```python
from build123d import *

# Parameters (mm, degrees)
BOSS_EXTRUDE1_DEPTH = 200.8
CUT_EXTRUDE3_DEPTH  = 36.191113799
SKETCH5_W           = 20
SKETCH5_H           = 5
SKETCH5_W_2         = 3
SKETCH5_H_2         = 20
SKETCH5_H_3         = 3
BOSS_EXTRUDE2_DEPTH = 5


with BuildPart() as part:
    # Sketch2 → Boss-Extrude1 (new body)
    with BuildSketch(Plane.XY.offset(2)):
        Polygon((22.534227339, 12.285835046), (24.243029584, 7.58689954), (-64.096957923, -24.53858267), (-65.805760168, -19.839647165), align=None)
    extrude(amount=BOSS_EXTRUDE1_DEPTH)

    # Sketch4 → Cut-Extrude3 (cut, through all)
    with BuildSketch(Plane(origin=(0.394814778, -1.085678102, 0), x_dir=(-0.939787101, -0.341760449, 0), z_dir=(0.341760449, -0.939787101, 0))):
        Polygon((19.52381131, -2), (23.72381131, -2), (23.72381131, -6), (25.42381131, -6), (25.42381131, -8.8), (23.72381131, -8.8), (23.72381131, -18.8), (19.52381131, -18.8), (19.52381131, -8.8), (17.82381131, -8.8), (17.82381131, -6), (19.52381131, -6), align=None)
        Polygon((-25.37618869, -54.3), (-25.37618869, -50.1), (-21.37618869, -50.1), (-21.37618869, -48.4), (-18.57618869, -48.4), (-18.57618869, -50.1), (-8.57618869, -50.1), (-8.57618869, -54.3), (-18.57618869, -54.3), (-18.57618869, -56), (-21.37618869, -56), (-21.37618869, -54.3), align=None)
        Polygon((23.72381131, -202.8), (19.52381131, -202.8), (19.52381131, -198.8), (17.82381131, -198.8), (17.82381131, -196), (19.52381131, -196), (19.52381131, -186), (23.72381131, -186), (23.72381131, -196), (25.42381131, -196), (25.42381131, -198.8), (23.72381131, -198.8), align=None)
        Polygon((-21.37618869, -154.7), (-21.37618869, -156.4), (-18.57618869, -156.4), (-18.57618869, -154.7), (-8.57618869, -154.7), (-8.57618869, -150.5), (-18.57618869, -150.5), (-18.57618869, -148.8), (-21.37618869, -148.8), (-21.37618869, -150.5), (-25.37618869, -150.5), (-25.37618869, -154.7), align=None)
        Polygon((68.62381131, -150.5), (68.62381131, -154.7), (64.62381131, -154.7), (64.62381131, -156.4), (61.82381131, -156.4), (61.82381131, -154.7), (51.82381131, -154.7), (51.82381131, -150.5), (61.82381131, -150.5), (61.82381131, -148.8), (64.62381131, -148.8), (64.62381131, -150.5), align=None)
        Polygon((64.62381131, -50.1), (64.62381131, -48.4), (61.82381131, -48.4), (61.82381131, -50.1), (51.82381131, -50.1), (51.82381131, -54.3), (61.82381131, -54.3), (61.82381131, -56), (64.62381131, -56), (64.62381131, -54.3), (68.62381131, -54.3), (68.62381131, -50.1), align=None)
    extrude(amount=-CUT_EXTRUDE3_DEPTH, mode=Mode.SUBTRACT)

    # Sketch5 → Boss-Extrude2 (add)
    with BuildSketch(Plane(origin=(0.394814778, -1.085678102, 0), x_dir=(0.939787101, 0.341760449, 0), z_dir=(0.341760449, -0.939787101, 0))):
        with Locations((2.92618869, -0.5)):
            Rectangle(SKETCH5_W, SKETCH5_H)
        with Locations((-46.17381131, -0.5)):
            Rectangle(SKETCH5_W, SKETCH5_H)
        with Locations((26.87618869, 102.4)):
            Rectangle(SKETCH5_W_2, SKETCH5_H_2)
        with Locations((26.87618869, 178.75)):
            Rectangle(SKETCH5_W_2, SKETCH5_H_2)
        with Locations((2.92618869, 204.3)):
            Rectangle(SKETCH5_W, SKETCH5_H_3)
        with Locations((-46.17381131, 204.3)):
            Rectangle(SKETCH5_W, SKETCH5_H_3)
    extrude(amount=-BOSS_EXTRUDE2_DEPTH)


solid = part.part
```
Can you work these out from the model? Positions are in its coordinate system, mm. A direction names the side the tool comes from. Round coordinates to 2 decimals unless told otherwise and drop trailing zeros. Loops run counter-clockwise (first coordinate to the right, second up) from the corner with the lowest first, then second, coordinate; pieces in that order, holes last. Notation, with made-up numbers: M 52.25,69.25 L 79.25,69.25 A16 cw 79.25,97.25 Z; hole C 16.25,45.25 d8. An arc over 180 degrees is marked long. Write item = value, one per line. Start each with the question number.
(1) Which directions (+Z, -Z, +X, -X, +Y, -Y) give clear straight access to the entire face, cutting with the end or side of a thin tool? Please do faces 5 (the face through (-49.15, -16.48, 152.63)), 6 (the face through (18, 8, 56)), 7 (the face through (7.6, 4.2, 152.6)).
(2) If we mould it in two halves opening along Z, with no side actions, what happens to faces 1 (the face through (-21, -6, 186)), 2 (the face through (-60, -20, 48.4)), 3 (the face through (-54, -18, 50.1)), 4 (the face through (-64.94, -22.22, 25.71))? For each: released by +Z, released by -Z, zero draft, split by the parting line, or undercut.
(3) I'm going to push flat-ended pins straight in: P1, Ø4.5, axis at x = 21, y = 8, coming from the +Z side; P2, Ø1, axis at x = -24.5, y = -8.5, coming from the -Z side; P3, Ø1.5, axis at x = -20, z = 77, coming from the -Y side; P4, Ø9, axis at x = -55.5, y = -18.5, coming from the -Z side. Where does each tip first touch, or does it pass through?
(4) Suppose I cut it at C-C on x = -31.5. Write out the boundary of the cut face in (y, z).
(5) Suppose I cut it at A-A on z = 61. Write out the boundary of the cut face in (x, y), plus the area to 3 significant figures.
(6) I need wall thicknesses on line 1 along Z through (x, y) = (11.5, 3); line 2 along Y through (x, z) = (-2.5, 116.5); line 3 along Y through (x, z) = (-12, 98.5). Which ranges of each line are inside material? Lowest first, please.
(7) Suppose I cut it at B-B on x = -4. Write out the boundary of the cut face in (y, z).
Answer block:
q1.face_5 = -X, -Y
q1.face_6 = none
q1.face_7 = +X, +Y
q2.face_1 = released by +Z
q2.face_2 = undercut
q2.face_3 = undercut
q2.face_4 = zero draft
q3.P1 = 202.8
q3.P2 = 2
q3.P3 = -8.78
q3.P4 = -3
q4.outline = M -12.68,2 L -7.36,2 L -7.36,202.8 L -12.68,202.8 Z
q5.outline = M -65.81,-19.84 L -64.1,-24.54 L 24.24,7.59 L 22.53,12.29 Z
q5.area = 470 mm²
q6.line_1 = -3 to 50.1, 54.3 to 150.5, 154.7 to 205.8
q6.line_2 = -2.14 to 3.18
q6.line_3 = -5.59 to -0.27
q7.outline = M -2.68,-3 L 2.64,-3 L 2.64,205.8 L -2.68,205.8 Z
